from build123d import *

# Parameters (mm, degrees)
F0_W     = 100
F0_H     = 40
F1_DEPTH = 10
F2_R     = 2
F3_DEPTH = 10.001
F4_R     = 2
F5_DEPTH = 10.001


with BuildPart() as f1:
    # F0 (on Right) → F1 (new body)
    with BuildSketch(Plane.YZ):
        Rectangle(F0_W, F0_H)
    extrude(amount=F1_DEPTH)

    # F2 (on face) → F3 (cut, through all)
    with BuildSketch(Plane.YZ.offset(10)):
        with Locations((-15, 15)):
            Circle(F2_R)
        with Locations((15, 15)):
            Circle(F2_R)
        with Locations((-15, -15)):
            Circle(F2_R)
        with Locations((15, -15)):
            Circle(F2_R)
    extrude(amount=-F3_DEPTH, mode=Mode.SUBTRACT)

    # F4 (on face) → F5 (cut, through all)
    with BuildSketch(Plane.YZ.offset(10)):
        with Locations((-41, 0)):
            Circle(F4_R)
        with Locations((41, 0)):
            Circle(F4_R)
    extrude(amount=-F5_DEPTH, mode=Mode.SUBTRACT)


solid = f1.part
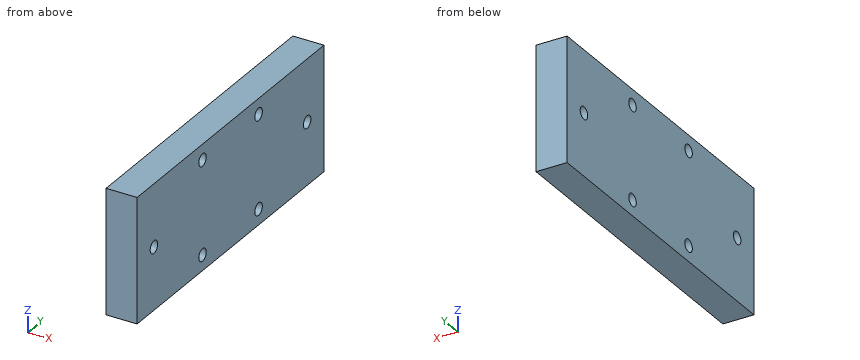
CAD build for the part. Positions are in the model's coordinates, mm. Give positions to 0.01 mm unless a question says otherwise; leave off trailing zeros. Write each loop counter-clockwise with the first axis right and the second up, starting at its lowest first coordinate (ties: lowest second). Pieces come first, ordered by that corner, then holes. Notation, with made-up numbers: (18, 60) - (35, 60) arc R17 cw to (35, 71) - close; hole circle Ø2 at (76.25, 61). An arc over 180 degrees is marked (long way). Put each result on its own line as item: value.
(1) Saw through at C-C (x = 1.5). List the corners of the cut face in (y, z).
Working result:
outline: (-50, -20) - (50, -20) - (50, 20) - (-50, 20) - close; hole circle Ø4 at (-41, 0); hole circle Ø4 at (-15, -15); hole circle Ø4 at (-15, 15); hole circle Ø4 at (15, -15); hole circle Ø4 at (15, 15); hole circle Ø4 at (41, 0)
(2) Saw through at D-D (y = -15). List the corners of the cut face in (x, z).
Working result:
outline: (0, -20) - (10, -20) - (10, -17) - (0, -17) - close; (0, -13) - (10, -13) - (10, 13) - (0, 13) - close; (0, 17) - (10, 17) - (10, 20) - (0, 20) - close
(3) Saw through at A-A (z = 0). List the corners of the cut face in (x, y), then the cut area to 3 significant figures.
Working result:
outline: (0, -50) - (10, -50) - (10, -43) - (0, -43) - close; (0, -39) - (10, -39) - (10, 39) - (0, 39) - close; (0, 43) - (10, 43) - (10, 50) - (0, 50) - close
area: 920 mm^2
(4) Drop flat-ended pins along their axis: pin 1 Ø6.5 at (y, z) = (15, -15) entering from +X; pin 2 Ø3 at (y, z) = (-41, 0) entering from -X. Give the stop position or say it passes through.
Working result:
pin 1: x = 10
pin 2: through
(5) Saw through at B-B (y = -41). List the corners of the cut face in (x, z), then the cut area to 3 significant figures.
Working result:
outline: (0, -20) - (10, -20) - (10, -2) - (0, -2) - close; (0, 2) - (10, 2) - (10, 20) - (0, 20) - close
area: 360 mm^2
(6) Wall check: L1, parallel to Z at x = 5, y = 15; L2, parallel to Z at x = 4, y = -41; L3, parallel to Z at x = 7.75, y = -39.5. Give the ranges that are in metal, low to high.
Working result:
L1: -20 to -17, -13 to 13, 17 to 20
L2: -20 to -2, 2 to 20
L3: -20 to -1.32, 1.32 to 20
